```python
from build123d import *

# Parameters (mm, degrees)
F0_R     = 28.486326
F0_R_2   = 2.325
F1_DEPTH = 5


with BuildPart() as f1:
    # F0 (on Top) → F1 (new body)
    with BuildSketch(Plane.XY):
        Circle(F0_R)
        with Locations((-16.043124, -19.119451)):
            Circle(F0_R_2, mode=Mode.SUBTRACT)
        with Locations((-8.536368, -23.453478)):
            Circle(F0_R_2, mode=Mode.SUBTRACT)
        with Locations((-12.45077, -14.83825)):
            Circle(F0_R_2, mode=Mode.SUBTRACT)
        with Locations((-6.624916, -18.201808)):
            Circle(F0_R_2, mode=Mode.SUBTRACT)
        with Locations((-21.614842, -12.479335)):
            Circle(F0_R_2, mode=Mode.SUBTRACT)
        with Locations((-16.774877, -9.68498)):
            Circle(F0_R_2, mode=Mode.SUBTRACT)
        with Locations((-24.579492, -4.334028)):
            Circle(F0_R_2, mode=Mode.SUBTRACT)
        with Locations((-19.075687, -3.363558)):
            Circle(F0_R_2, mode=Mode.SUBTRACT)
        with Locations((0, -24.95867)):
            Circle(F0_R_2, mode=Mode.SUBTRACT)
        with Locations((8.536368, -23.453478)):
            Circle(F0_R_2, mode=Mode.SUBTRACT)
        with Locations((0, -19.36996)):
            Circle(F0_R_2, mode=Mode.SUBTRACT)
        with Locations((6.624916, -18.201808)):
            Circle(F0_R_2, mode=Mode.SUBTRACT)
        with Locations((12.45077, -14.83825)):
            Circle(F0_R_2, mode=Mode.SUBTRACT)
        with Locations((16.043124, -19.119451)):
            Circle(F0_R_2, mode=Mode.SUBTRACT)
        with Locations((16.774877, -9.68498)):
            Circle(F0_R_2, mode=Mode.SUBTRACT)
        with Locations((21.614842, -12.479335)):
            Circle(F0_R_2, mode=Mode.SUBTRACT)
        with Locations((19.075687, -3.363558)):
            Circle(F0_R_2, mode=Mode.SUBTRACT)
        with Locations((24.579492, -4.334028)):
            Circle(F0_R_2, mode=Mode.SUBTRACT)
        with Locations((-24.579492, 4.334028)):
            Circle(F0_R_2, mode=Mode.SUBTRACT)
        with Locations((-19.075687, 3.363558)):
            Circle(F0_R_2, mode=Mode.SUBTRACT)
        with Locations((-21.614842, 12.479335)):
            Circle(F0_R_2, mode=Mode.SUBTRACT)
        with Locations((-16.774877, 9.68498)):
            Circle(F0_R_2, mode=Mode.SUBTRACT)
        with Locations((-16.043124, 19.119451)):
            Circle(F0_R_2, mode=Mode.SUBTRACT)
        with Locations((-12.45077, 14.83825)):
            Circle(F0_R_2, mode=Mode.SUBTRACT)
        with Locations((-6.624916, 18.201808)):
            Circle(F0_R_2, mode=Mode.SUBTRACT)
        with Locations((-8.536368, 23.453478)):
            Circle(F0_R_2, mode=Mode.SUBTRACT)
        with BuildLine():
            ThreePointArc((13.999521, 0.11578), (13.99988, 0.05789), (14, 0))
            ThreePointArc((14, 0), (13.99988, -0.05789), (13.999521, -0.11578))
            ThreePointArc((13.999521, -0.11578), (15.504722, -0.863875), (16.112309, -2.431074))
            ThreePointArc((16.112309, -2.431074), (15.206489, -4.272691), (13.194846, -4.679321))
            ThreePointArc((13.194846, -4.679321), (13.155697, -4.788282), (13.115648, -4.896915))
            ThreePointArc((13.115648, -4.896915), (14.087819, -5.754835), (14.449356, -7))
            ThreePointArc((14.449356, -7), (13.202183, -9.060076), (10.798677, -8.910027))
            ThreePointArc((10.798677, -8.910027), (10.724622, -8.999027), (10.649834, -9.087411))
            ThreePointArc((10.649834, -9.087411), (11.148881, -9.839326), (11.324027, -10.724622))
            ThreePointArc((11.324027, -10.724622), (9.702751, -12.940564), (7.100029, -12.066051))
            ThreePointArc((7.100029, -12.066051), (7, -12.124356), (6.899493, -12.181831))
            ThreePointArc((6.899493, -12.181831), (7.059206, -12.657169), (7.113282, -13.155697))
            ThreePointArc((7.113282, -13.155697), (5.096521, -15.460174), (2.545012, -13.766732))
            ThreePointArc((2.545012, -13.766732), (2.431074, -13.787309), (2.316971, -13.806942))
            ThreePointArc((2.316971, -13.806942), (2.322992, -13.903388), (2.325, -14))
            ThreePointArc((2.325, -14), (-0.096612, -16.322992), (-2.316971, -13.806942))
            ThreePointArc((-2.316971, -13.806942), (-2.431074, -13.787309), (-2.545012, -13.766732))
            ThreePointArc((-2.545012, -13.766732), (-5.583479, -15.340482), (-6.899493, -12.181831))
            ThreePointArc((-6.899493, -12.181831), (-7, -12.124356), (-7.100029, -12.066051))
            ThreePointArc((-7.100029, -12.066051), (-10.493508, -12.505676), (-10.649834, -9.087411))
            ThreePointArc((-10.649834, -9.087411), (-10.724622, -8.999027), (-10.798677, -8.910027))
            ThreePointArc((-10.798677, -8.910027), (-14.137865, -8.1625), (-13.115648, -4.896915))
            ThreePointArc((-13.115648, -4.896915), (-13.155697, -4.788282), (-13.194846, -4.679321))
            ThreePointArc((-13.194846, -4.679321), (-16.076987, -2.834807), (-13.999521, -0.11578))
            ThreePointArc((-13.999521, -0.11578), (-14, 0), (-13.999521, 0.11578))
            ThreePointArc((-13.999521, 0.11578), (-16.076987, 2.834807), (-13.194846, 4.679321))
            ThreePointArc((-13.194846, 4.679321), (-13.155697, 4.788282), (-13.115648, 4.896915))
            ThreePointArc((-13.115648, 4.896915), (-14.137865, 8.1625), (-10.798677, 8.910027))
            ThreePointArc((-10.798677, 8.910027), (-10.724622, 8.999027), (-10.649834, 9.087411))
            ThreePointArc((-10.649834, 9.087411), (-10.493508, 12.505676), (-7.100029, 12.066051))
            ThreePointArc((-7.100029, 12.066051), (-7, 12.124356), (-6.899493, 12.181831))
            ThreePointArc((-6.899493, 12.181831), (-5.583479, 15.340482), (-2.545012, 13.766732))
            ThreePointArc((-2.545012, 13.766732), (-2.431074, 13.787309), (-2.316971, 13.806942))
            ThreePointArc((-2.316971, 13.806942), (-0.096612, 16.322992), (2.325, 14))
            ThreePointArc((2.325, 14), (2.322992, 13.903388), (2.316971, 13.806942))
            ThreePointArc((2.316971, 13.806942), (2.431074, 13.787309), (2.545012, 13.766732))
            ThreePointArc((2.545012, 13.766732), (5.096521, 15.460174), (7.113282, 13.155697))
            ThreePointArc((7.113282, 13.155697), (7.059206, 12.657169), (6.899493, 12.181831))
            ThreePointArc((6.899493, 12.181831), (7, 12.124356), (7.100029, 12.066051))
            ThreePointArc((7.100029, 12.066051), (9.702751, 12.940564), (11.324027, 10.724622))
            ThreePointArc((11.324027, 10.724622), (11.148881, 9.839326), (10.649834, 9.087411))
            ThreePointArc((10.649834, 9.087411), (10.724622, 8.999027), (10.798677, 8.910027))
            ThreePointArc((10.798677, 8.910027), (13.202183, 9.060076), (14.449356, 7))
            ThreePointArc((14.449356, 7), (14.087819, 5.754835), (13.115648, 4.896915))
            ThreePointArc((13.115648, 4.896915), (13.155697, 4.788282), (13.194846, 4.679321))
            ThreePointArc((13.194846, 4.679321), (15.206489, 4.272691), (16.112309, 2.431074))
            ThreePointArc((16.112309, 2.431074), (15.504722, 0.863875), (13.999521, 0.11578))
        make_face(mode=Mode.SUBTRACT)
        with Locations((19.075687, 3.363558)):
            Circle(F0_R_2, mode=Mode.SUBTRACT)
        with Locations((24.579492, 4.334028)):
            Circle(F0_R_2, mode=Mode.SUBTRACT)
        with Locations((16.774877, 9.68498)):
            Circle(F0_R_2, mode=Mode.SUBTRACT)
        with Locations((21.614842, 12.479335)):
            Circle(F0_R_2, mode=Mode.SUBTRACT)
        with Locations((0, 19.36996)):
            Circle(F0_R_2, mode=Mode.SUBTRACT)
        with Locations((6.624916, 18.201808)):
            Circle(F0_R_2, mode=Mode.SUBTRACT)
        with Locations((12.45077, 14.83825)):
            Circle(F0_R_2, mode=Mode.SUBTRACT)
        with Locations((0, 24.95867)):
            Circle(F0_R_2, mode=Mode.SUBTRACT)
        with Locations((8.536368, 23.453478)):
            Circle(F0_R_2, mode=Mode.SUBTRACT)
        with Locations((16.043124, 19.119451)):
            Circle(F0_R_2, mode=Mode.SUBTRACT)
        with BuildLine():
            ThreePointArc((13.999521, -0.11578), (13.99988, -0.05789), (14, 0))
            ThreePointArc((14, 0), (13.99988, 0.05789), (13.999521, 0.11578))
            ThreePointArc((13.999521, 0.11578), (11.497631, 2.027342), (13.194846, 4.679321))
            ThreePointArc((13.194846, 4.679321), (13.155697, 4.788282), (13.115648, 4.896915))
            ThreePointArc((13.115648, 4.896915), (10.110847, 5.8375), (10.798677, 8.910027))
            ThreePointArc((10.798677, 8.910027), (10.724622, 8.999027), (10.649834, 9.087411))
            ThreePointArc((10.649834, 9.087411), (7.504545, 8.943569), (7.100029, 12.066051))
            ThreePointArc((7.100029, 12.066051), (7, 12.124356), (6.899493, 12.181831))
            ThreePointArc((6.899493, 12.181831), (3.993085, 10.970911), (2.545012, 13.766732))
            ThreePointArc((2.545012, 13.766732), (2.431074, 13.787309), (2.316971, 13.806942))
            ThreePointArc((2.316971, 13.806942), (0, 11.675), (-2.316971, 13.806942))
            ThreePointArc((-2.316971, 13.806942), (-2.431074, 13.787309), (-2.545012, 13.766732))
            ThreePointArc((-2.545012, 13.766732), (-2.483805, 13.463935), (-2.463282, 13.155697))
            ThreePointArc((-2.463282, 13.155697), (-4.289754, 10.884773), (-6.899493, 12.181831))
            ThreePointArc((-6.899493, 12.181831), (-7, 12.124356), (-7.100029, 12.066051))
            ThreePointArc((-7.100029, 12.066051), (-6.783085, 11.428346), (-6.674027, 10.724622))
            ThreePointArc((-6.674027, 10.724622), (-8.113731, 8.574767), (-10.649834, 9.087411))
            ThreePointArc((-10.649834, 9.087411), (-10.724622, 8.999027), (-10.798677, 8.910027))
            ThreePointArc((-10.798677, 8.910027), (-10.064279, 8.077827), (-9.799356, 7))
            ThreePointArc((-9.799356, 7), (-10.879191, 5.036536), (-13.115648, 4.896915))
            ThreePointArc((-13.115648, 4.896915), (-13.155697, 4.788282), (-13.194846, 4.679321))
            ThreePointArc((-13.194846, 4.679321), (-11.945692, 3.850255), (-11.462309, 2.431074))
            ThreePointArc((-11.462309, 2.431074), (-12.220109, 0.713661), (-13.999521, 0.11578))
            ThreePointArc((-13.999521, 0.11578), (-14, 0), (-13.999521, -0.11578))
            ThreePointArc((-13.999521, -0.11578), (-12.220109, -0.713661), (-11.462309, -2.431074))
            ThreePointArc((-11.462309, -2.431074), (-11.945692, -3.850255), (-13.194846, -4.679321))
            ThreePointArc((-13.194846, -4.679321), (-13.155697, -4.788282), (-13.115648, -4.896915))
            ThreePointArc((-13.115648, -4.896915), (-10.879191, -5.036536), (-9.799356, -7))
            ThreePointArc((-9.799356, -7), (-10.064279, -8.077827), (-10.798677, -8.910027))
            ThreePointArc((-10.798677, -8.910027), (-10.724622, -8.999027), (-10.649834, -9.087411))
            ThreePointArc((-10.649834, -9.087411), (-8.113731, -8.574767), (-6.674027, -10.724622))
            ThreePointArc((-6.674027, -10.724622), (-6.783085, -11.428346), (-7.100029, -12.066051))
            ThreePointArc((-7.100029, -12.066051), (-7, -12.124356), (-6.899493, -12.181831))
            ThreePointArc((-6.899493, -12.181831), (-4.289754, -10.884773), (-2.463282, -13.155697))
            ThreePointArc((-2.463282, -13.155697), (-2.483805, -13.463935), (-2.545012, -13.766732))
            ThreePointArc((-2.545012, -13.766732), (-2.431074, -13.787309), (-2.316971, -13.806942))
            ThreePointArc((-2.316971, -13.806942), (0, -11.675), (2.316971, -13.806942))
            ThreePointArc((2.316971, -13.806942), (2.431074, -13.787309), (2.545012, -13.766732))
            ThreePointArc((2.545012, -13.766732), (3.993085, -10.970911), (6.899493, -12.181831))
            ThreePointArc((6.899493, -12.181831), (7, -12.124356), (7.100029, -12.066051))
            ThreePointArc((7.100029, -12.066051), (7.504545, -8.943569), (10.649834, -9.087411))
            ThreePointArc((10.649834, -9.087411), (10.724622, -8.999027), (10.798677, -8.910027))
            ThreePointArc((10.798677, -8.910027), (10.110847, -5.8375), (13.115648, -4.896915))
            ThreePointArc((13.115648, -4.896915), (13.155697, -4.788282), (13.194846, -4.679321))
            ThreePointArc((13.194846, -4.679321), (11.497631, -2.027342), (13.999521, -0.11578))
        make_face()
    extrude(amount=F1_DEPTH)


solid = f1.part
```
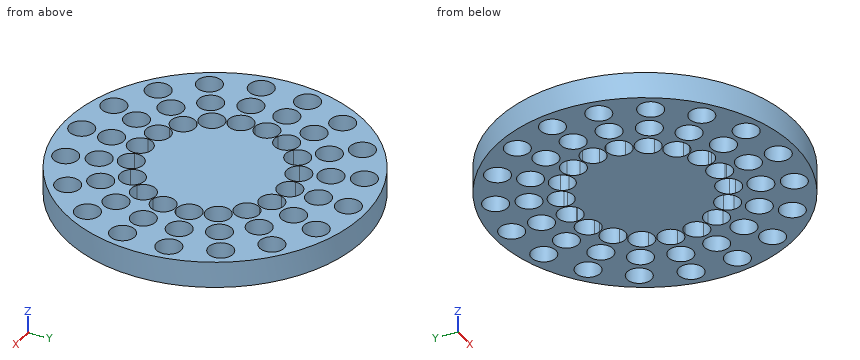
Build history of the part. All positions in model axes, mm. Round coordinates to 2 decimals unless told otherwise and drop trailing zeros. Order: outer loops, then holes, each group sorted by start corner. A loop starts at its lowest first (then second) coordinate and runs counter-clockwise, first axis right, second up. Notation, with made-up numbers: (49, 38.5) - (103, 38.5) arc R23 ccw to (103, 47.5) - close; hole circle Ø10 at (89, 82.5). An arc over 180 degrees is marked (long way). Use a Markdown table: item, result.
1) Saw through at B-B on x = 20.5. Write the cut outline in (y, z), and give its area (3 significant figures).
Recorded:
| item | result |
|---|---|
| outline | (-19.78, 0) - (-14.52, 0) - (-14.52, 5) - (-19.78, 5) - close; (-10.44, 0) - (-5.2, 0) - (-5.2, 5) - (-10.44, 5) - close; (-1.53, 0) - (1.53, 0) - (1.53, 5) - (-1.53, 5) - close; (5.2, 0) - (10.44, 0) - (10.44, 5) - (5.2, 5) - close; (14.52, 0) - (19.78, 0) - (19.78, 5) - (14.52, 5) - close |
| area | 120 mm² |
2) Wall check: L1, parallel to X at y = -24.5, z = 2.2; L2, parallel to X at y = -21.5, z = 2.6; L3, parallel to Y at x = 3, z = 4.7. Give the ranges that are in metal, low to high.
Recorded:
| item | result |
|---|---|
| L1 | x = -14.53 to -10.61, -6.46 to -2.28, 2.28 to 6.46, 10.61 to 14.53 |
| L2 | x = -18.69 to -9.8, -7.28 to -0.93, 0.93 to 7.28, 9.8 to 18.69 |
| L3 | y = -28.33 to -14.64, -11.67 to 11.67, 14.64 to 28.33 |
3) Saw through at A-A on x = -1.5. Write the cut outline in (y, z), and give its area (3 significant figures).
Recorded:
| item | result |
|---|---|
| outline | (-28.45, 0) - (-26.74, 0) - (-26.74, 5) - (-28.45, 5) - close; (-23.18, 0) - (-21.15, 0) - (-21.15, 5) - (-23.18, 5) - close; (-17.59, 0) - (-15.78, 0) - (-15.78, 5) - (-17.59, 5) - close; (-12.22, 0) - (12.22, 0) - (12.22, 5) - (-12.22, 5) - close; (15.78, 0) - (17.59, 0) - (17.59, 5) - (15.78, 5) - close; (21.15, 0) - (23.18, 0) - (23.18, 5) - (21.15, 5) - close; (26.74, 0) - (28.45, 0) - (28.45, 5) - (26.74, 5) - close |
| area | 178 mm² |
4) Saw through at C-C on z = 3.35. Give the number of separate pieces and of enclosed holes in the cut face, and give its area (3 significant figures).
Recorded:
| item | result |
|---|---|
| separate pieces | 1 |
| enclosed holes | 54 |
| area | 1,630 mm² |
5) Flat gauge pins, fed straight in: pin 1 Ø3 at (x, y) = (-13.79, 2.43) entering from +Z; pin 2 Ø1.5 at (y, z) = (13, 4) entering from +X; pin 3 Ø1.5 at (x, z) = (20.5, 0.5) entering from +Y. Where does each tip first touch, or does it go through?
Recorded:
| item | result |
|---|---|
| pin 1 | passes through |
| pin 2 | stops at x = 25.72 |
| pin 3 | stops at y = 20.53 |
